from build123d import *

# Parameters (mm, degrees)
SKETCH4_R          = 0.8
CUT_EXTRUDE1_DEPTH = 13.861305914


with BuildPart() as part:
    # Sketch3 → Revolve19 (revolve)
    with BuildSketch(Plane.XY):
        Polygon((295.058388758, -144.573704322), (295.058388758, -144.073704322), (305.058388758, -144.073704322), (305.058388758, -143.073704322), (261.558388758, -143.073704322), (261.558388758, -144.323704322), (261.558388758, -148.073704322), (263.058388758, -148.073704322), (263.058388758, -144.573704322), align=None)
    revolve(axis=Axis((263.058388758, -148.573704322, 0), (1, 0, 0)))

    # Sketch4 → Cut-Extrude1 (cut, through all)
    with BuildSketch(Plane(origin=(0, -26.447590039, -53.851341485), x_dir=(1, 0, 0), z_dir=(0, 0.440827333, 0.897591924))):
        with Locations((298.024345503, -133.358557166)):
            Circle(SKETCH4_R)
    extrude(amount=-CUT_EXTRUDE1_DEPTH, mode=Mode.SUBTRACT)


solid = part.part
Source: CAD feature listing. Evaluate the final solid. Frame: model axes, mm. A direction names the side the tool comes from. Coordinates: 2 decimals unless noted, no trailing zeros. Loops run counter-clockwise (first coordinate to the right, second up) from the corner with the lowest first, then second, coordinate; pieces in that order, holes last. Notation, with made-up numbers: M -12,10 L 38,10 A24 ccw 38,44 Z; hole C -27,46.5 d9. An arc over 180 degrees is marked long. Answer in a Markdown table with one row per item.
Q1. Section C-C on z = 2.5. Return the cut outline in (x, y), plus the area to 3 significant figures.
Answers below:
| item | result |
|---|---|
| outline | M 261.56,-153.47 L 305.06,-153.47 L 305.06,-152.32 L 295.06,-152.32 L 295.06,-151.7 L 263.06,-151.7 L 263.06,-145.45 L 295.06,-145.45 L 295.06,-144.83 L 305.06,-144.83 L 305.06,-143.67 L 261.56,-143.67 Z |
| area | 152 mm^2 |
Q2. Set-up query: faces 1 (the cylindrical face through (262.32, -148.11, -0.19)), 2 (the cylindrical face through (300.128, -149.549, -4.393)). Return all of +Z, -Z, +X, -X, +Y, -Y with unobstructed straight access to the full face (end or side cutting, diameter ignored); none if empty.
Answers below:
| item | result |
|---|---|
| face 1 | +X, -X |
| face 2 | +X |
Q3. Section A-A on z = 0. Return the cut outline in (x, y).
Answers below:
| item | result |
|---|---|
| outline | M 261.56,-154.07 L 305.06,-154.07 L 305.06,-153.07 L 295.06,-153.07 L 295.06,-152.57 L 263.06,-152.57 L 263.06,-149.07 L 261.56,-149.07 Z; M 261.56,-148.07 L 263.06,-148.07 L 263.06,-144.57 L 295.06,-144.57 L 295.06,-144.07 L 305.06,-144.07 L 305.06,-143.07 L 261.56,-143.07 Z |
Q4. First-contact query: pin 1 (6 mm diameter, centred on x = 279.5, z = 1.5, fed in from +Y); pin 2 (4.5 mm diameter, centred on y = -149.5, z = 0.5, fed in from +X); pin 3 (3 mm diameter, centred on x = 267, z = -4, fed in from -Y). Flat tips, straight axial feed; report the tip coordinate or a pass-through.
Answers below:
| item | result |
|---|---|
| pin 1 | stops at y = -143.07 |
| pin 2 | stops at x = 263.06 |
| pin 3 | stops at y = -153.47 |
Q5. Draft query along Y for faces 3 (the cylindrical face through (283.004, -143.328, 1.652)), 4 (the flat face through (263.058, -149, -1)), 5 (the flat face through (261.558, -147, 0)). Return one class per face: pulls with the +Y half, pulls with the -Y half, needs draft (parallel to the pull), parting line crosses it, or undercut.
Answers below:
| item | result |
|---|---|
| face 3 | parting line crosses it |
| face 4 | undercut |
| face 5 | needs draft |
Q6. Section B-B on x = 283. Return the cut outline in (y, z).
Answers below:
| item | result |
|---|---|
| outline | C -148.57,0 d11; hole C -148.57,0 d8 |
Q7. Ray query, probe 1 along X at (y, z) = (-150.5, 0.75); probe 2 along Z at (x, y) = (281, -146); probe 3 along Z at (x, y) = (266.5, -148.5). Return the intervals inside material, ascending. Write a range as from..to.
Answers below:
| item | result |
|---|---|
| probe 1 | x = 261.56..263.06 |
| probe 2 | z = -4.86..-3.06, 3.06..4.86 |
| probe 3 | z = -5.5..-4, 4..5.5 |
